```python
from build123d import *

# Parameters (mm, degrees)
F0_R     = 37.5
F0_R_2   = 5.5
F1_DEPTH = 7


with BuildPart() as f1:
    # F0 (on Top) → F1 (new body)
    with BuildSketch(Plane.XY):
        Circle(F0_R)
        with BuildLine():
            ThreePointArc((-2.377026, -34.418015), (-14.293428, -31.399808), (-24.395184, -24.395184))
            ThreePointArc((-24.395184, -24.395184), (-10.462875, -20.649823), (-6.717514, -6.717514))
            ThreePointArc((-6.717514, -6.717514), (-4.251838, -8.495403), (-1.350829, -9.403471))
            ThreePointArc((-1.350829, -9.403471), (1.909461, -22.065542), (-2.377026, -34.418015))
        make_face(mode=Mode.SUBTRACT)
        with BuildLine():
            ThreePointArc((-26.018023, -22.656401), (-32.309997, -12.096037), (-34.5, 0))
            ThreePointArc((-34.5, 0), (-22, -7.20326), (-9.5, 0))
            ThreePointArc((-9.5, 0), (-9.013661, -3.000653), (-7.604438, -5.694078))
            ThreePointArc((-7.604438, -5.694078), (-14.252502, -16.952887), (-26.018023, -22.656401))
        make_face(mode=Mode.SUBTRACT)
        with BuildLine():
            ThreePointArc((22.656401, -26.018023), (12.096037, -32.309997), (0, -34.5))
            ThreePointArc((0, -34.5), (7.20326, -22), (0, -9.5))
            ThreePointArc((0, -9.5), (3.000653, -9.013661), (5.694078, -7.604438))
            ThreePointArc((5.694078, -7.604438), (16.952887, -14.252502), (22.656401, -26.018023))
        make_face(mode=Mode.SUBTRACT)
        with BuildLine():
            ThreePointArc((9.403471, -1.350829), (22.065542, 1.909461), (34.418015, -2.377026))
            ThreePointArc((34.418015, -2.377026), (31.399808, -14.293428), (24.395184, -24.395184))
            ThreePointArc((24.395184, -24.395184), (20.649823, -10.462875), (6.717514, -6.717514))
            ThreePointArc((6.717514, -6.717514), (8.495403, -4.251838), (9.403471, -1.350829))
        make_face(mode=Mode.SUBTRACT)
        with BuildLine():
            ThreePointArc((-34.418015, 2.377026), (-31.399808, 14.293428), (-24.395184, 24.395184))
            ThreePointArc((-24.395184, 24.395184), (-20.649823, 10.462875), (-6.717514, 6.717514))
            ThreePointArc((-6.717514, 6.717514), (-8.495403, 4.251838), (-9.403471, 1.350829))
            ThreePointArc((-9.403471, 1.350829), (-22.065542, -1.909461), (-34.418015, 2.377026))
        make_face(mode=Mode.SUBTRACT)
        with BuildLine():
            ThreePointArc((-22.656401, 26.018023), (-12.096037, 32.309997), (0, 34.5))
            ThreePointArc((0, 34.5), (-7.20326, 22), (0, 9.5))
            ThreePointArc((0, 9.5), (-3.000653, 9.013661), (-5.694078, 7.604438))
            ThreePointArc((-5.694078, 7.604438), (-16.952887, 14.252502), (-22.656401, 26.018023))
        make_face(mode=Mode.SUBTRACT)
        Circle(F0_R_2, mode=Mode.SUBTRACT)
        with BuildLine():
            ThreePointArc((26.018023, 22.656401), (32.309997, 12.096037), (34.5, 0))
            ThreePointArc((34.5, 0), (22, 7.20326), (9.5, 0))
            ThreePointArc((9.5, 0), (9.013661, 3.000653), (7.604438, 5.694078))
            ThreePointArc((7.604438, 5.694078), (14.252502, 16.952887), (26.018023, 22.656401))
        make_face(mode=Mode.SUBTRACT)
        with BuildLine():
            ThreePointArc((2.377026, 34.418015), (14.293428, 31.399808), (24.395184, 24.395184))
            ThreePointArc((24.395184, 24.395184), (10.462875, 20.649823), (6.717514, 6.717514))
            ThreePointArc((6.717514, 6.717514), (4.251838, 8.495403), (1.350829, 9.403471))
            ThreePointArc((1.350829, 9.403471), (-1.909461, 22.065542), (2.377026, 34.418015))
        make_face(mode=Mode.SUBTRACT)
    extrude(amount=F1_DEPTH)


solid = f1.part
```
Geometry check sheet. Reference: the model listing, model coordinates, mm. A direction names the side the tool comes from. Round coordinates to 2 decimals unless told otherwise and drop trailing zeros. Order: outer loops, then holes, each group sorted by start corner. A loop starts at its lowest first (then second) coordinate and runs counter-clockwise, first axis right, second up. Notation, with made-up numbers: M 5,-29.75 L 24,-29.75 A26 cw 24,7.25 Z; hole C 12.5,-17.75 d4. An arc over 180 degrees is marked long. Answer as CSV lines item,"result".
1) Sectioned sample at A-A on z = 1.5. Give the number of separate pieces and of enclosed holes in the cut face, and give its area (3 significant figures).
Entries:
separate pieces,"1"
enclosed holes,"9"
area,"1,750 mm2"
2) Sectioned sample at C-C on x = -13. Record the cut outline in (y, z), and give its area (3 significant figures).
Entries:
outline,"M -35.17,0 L -31.96,0 L -31.96,7 L -35.17,7 Z; M -22.67,0 L -15.71,0 L -15.71,7 L -22.67,7 Z; M -4.06,0 L -0.41,0 L -0.41,7 L -4.06,7 Z; M 6.46,0 L 10.85,0 L 10.85,7 L 6.46,7 Z; M 31.96,0 L 35.17,0 L 35.17,7 L 31.96,7 Z"
area,"150 mm2"
3) Tool access check on faces 1 (the face through (0, 6, 0)), 2 (the face through (14.12, 16.83, 3.45)). Record the directions out of +Z, -Z, +X, -X, +Y, -Y that give a thin tool (end or side, any length) a straight path to the whole face; none if there is none.
Entries:
face 1,"-Z, +X, -X, +Y, -Y"
face 2,"+Z, -Z"
4) Gauge pin test, flat ends, axial feed: pin 1 Ø2 at (x, z) = (7.5, 6) entering from -Y; pin 2 Ø3 at (x, z) = (-30, 5.5) entering from -Y. Record the tip position at first contact, or that the pin passes through.
Entries:
pin 1,"y = -36.93"
pin 2,"y = -24.37"
5) Thickness scan on probe 1 along Y at (x, z) = (13.5, 3.5); probe 2 along X at (y, z) = (2, 3); probe 3 along X at (y, z) = (-19.5, 4.25). Record the ranges inside material, lowest first. Write a range as [from, to].
Entries:
probe 1,"[-34.99, -31.75], [-11.2, -6.56], [0.6, 4.44], [16.23, 22.97], [31.75, 34.99]"
probe 2,"[-37.45, -33.88], [-9.29, -5.12], [5.12, 9.29], [10.9, 33.1], [34.44, 37.45]"
probe 3,"[-32.03, -28.46], [-17.59, -9.43], [1.87, 6.99], [20.57, 24.83], [28.46, 32.03]"
6) Sectioned sample at B-B on y = 3.5. Record the cut outline in (x, z).
Entries:
outline,"M -37.34,0 L -34.32,0 L -34.32,7 L -37.34,7 Z; M -8.83,0 L -4.24,0 L -4.24,7 L -8.83,7 Z; M 4.24,0 L 8.83,0 L 8.83,7 L 4.24,7 Z; M 12.34,0 L 31.66,0 L 31.66,7 L 12.34,7 Z; M 34.32,0 L 37.34,0 L 37.34,7 L 34.32,7 Z"
